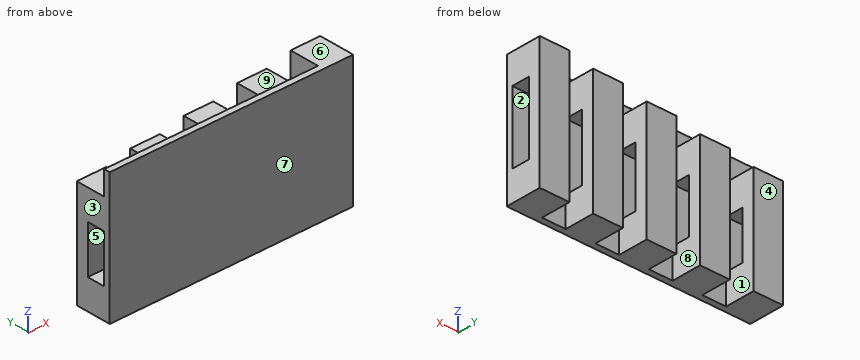
from build123d import *

# Parameters (mm, degrees)
SKETCH1_W            = 41
SKETCH1_H            = 22
BASE_DEPTH           = 1
SKETCH2_W            = 5
SKETCH2_H            = 5
LEGS_EXTRUSION_DEPTH = 5
SKETCH3_W            = 5
SKETCH3_H            = 2
BRIDGE1_DEPTH        = 8
SKETCH4_W            = 5
SKETCH4_H            = 2
BRIDGE2_DEPTH        = 9
SKETCH6_W            = 5
SKETCH6_H            = 2
BRIDGE3_DEPTH        = 10
SKETCH7_W            = 5
SKETCH7_H            = 2
BRIDGE4_DEPTH        = 11
SKETCH8_W            = 5
SKETCH8_H            = 2
BRIDGE5_DEPTH        = 12


with BuildPart() as part:
    # Sketch1 → Base (new body)
    with BuildSketch(Plane(origin=(0, 0, 0), x_dir=(1, 0, 0), z_dir=(0, 1, 0))):
        with Locations((20.5, 11)):
            Rectangle(SKETCH1_W, SKETCH1_H)
    extrude(amount=BASE_DEPTH)

    # Sketch2 → Legs_Extrusion (add)
    with BuildSketch(Plane(origin=(0, 1, 0), x_dir=(1, 0, 0), z_dir=(0, 1, 0))):
        with Locations((2.5, 19.5)):
            Rectangle(SKETCH2_W, SKETCH2_H)
        with Locations((2.5, 6.5)):
            Rectangle(SKETCH2_W, SKETCH2_H)
        with Locations((38.5, 2.5)):
            Rectangle(SKETCH2_W, SKETCH2_H)
        with Locations((38.5, 19.5)):
            Rectangle(SKETCH2_W, SKETCH2_H)
        with Locations((11.5, 19.5)):
            Rectangle(SKETCH2_W, SKETCH2_H)
        with Locations((11.5, 5.5)):
            Rectangle(SKETCH2_W, SKETCH2_H)
        with Locations((20.5, 19.5)):
            Rectangle(SKETCH2_W, SKETCH2_H)
        with Locations((29.5, 19.5)):
            Rectangle(SKETCH2_W, SKETCH2_H)
        with Locations((20.5, 4.5)):
            Rectangle(SKETCH2_W, SKETCH2_H)
        with Locations((29.5, 3.5)):
            Rectangle(SKETCH2_W, SKETCH2_H)
    extrude(amount=LEGS_EXTRUSION_DEPTH)

    # Sketch3 → bridge1 (add)
    with BuildSketch(Plane.XY.offset(-17)):
        with Locations((2.5, 5)):
            Rectangle(SKETCH3_W, SKETCH3_H)
    extrude(amount=BRIDGE1_DEPTH)

    # Sketch4 → bridge2 (add)
    with BuildSketch(Plane.XY.offset(-17)):
        with Locations((11.5, 5)):
            Rectangle(SKETCH4_W, SKETCH4_H)
    extrude(amount=BRIDGE2_DEPTH)

    # Sketch6 → bridge3 (add)
    with BuildSketch(Plane.XY.offset(-17)):
        with Locations((20.5, 5)):
            Rectangle(SKETCH6_W, SKETCH6_H)
    extrude(amount=BRIDGE3_DEPTH)

    # Sketch7 → bridge4 (add)
    with BuildSketch(Plane.XY.offset(-17)):
        with Locations((29.5, 5)):
            Rectangle(SKETCH7_W, SKETCH7_H)
    extrude(amount=BRIDGE4_DEPTH)

    # Sketch8 → bridge5 (add)
    with BuildSketch(Plane.XY.offset(-17)):
        with Locations((38.5, 5)):
            Rectangle(SKETCH8_W, SKETCH8_H)
    extrude(amount=BRIDGE5_DEPTH)


solid = part.part
Work out the finished part from the listing and answer in its coordinate system (mm). Face numbers are marked on the shaded views. A direction names the side the tool comes from. Coordinates: 2 decimals unless noted, no trailing zeros. Order: outer loops, then holes, each group sorted by start corner. A loop starts at its lowest first (then second) coordinate and runs counter-clockwise, first axis right, second up. Notation, with made-up numbers: (0.25, 66) - (21.25, 66) arc R14 cw to (21.25, 91) - close; hole circle Ø8 at (81.25, 80). An arc over 180 degrees is marked (long way). Put each result on its own line as item: value. Start each with the question number.
1) Flat-ended cylindrical pins translate along their axes: pin 1 (1.5 mm diameter, centred on x = 2, y = 2, fed in from +Z); pin 2 (2 mm diameter, centred on x = 24.5, z = -10.5, fed in from +Y); pin 3 (1.5 mm diameter, centred on x = 12.5, y = 2.5, fed in from +Z). Find the tip coordinate at first contact, or state that the pin passes through.
2) Find section B-B (x = 11). Give the vertices of the cut face in (y, z), plus the area to 3 significant figures.
3) Find the intervals of material crossed by line 1 (X direction, y = 4.45, z = -19.75); line 2 (Z direction, x = 9.5, y = 1.2); line 3 (Z direction, x = 20.5, y = 2.55), in increasing order. Write a range as from..to.
4) Find section C-C (z = -8.5). Give the vertices of the cut face in (x, y), plus the area to 3 significant figures.
5) Find section D-D (y = 4.8). Give the vertices of the cut face in (x, z).
6) For a pull along X with two mould halves and no side action, classify the marked faces 1, 2, 3 and 4 as released by +X, released by -X, zero draft, split by the parting line, or undercut.
7) Find section A-A (z = -16). Give the vertices of the cut face in (x, y), plus the area to 3 significant figures.
8) For the marked faces 5, 6, 7, 8 and 9, determine the directions among +Z, -Z, +X, -X, +Y, -Y from which every point of the face is accessible in a straight line to the end or side of a thin tool.
Results list:
1. pin 1: stops at z = -4
1. pin 2: stops at y = 1
1. pin 3: stops at z = -3
2. outline: (0, -22) - (6, -22) - (6, -3) - (1, -3) - (1, 0) - (0, 0) - close; hole (1, -17) - (4, -17) - (4, -8) - (1, -8) - close
2. area: 90.0 mm^2
3. line 1: x = 0..5, 9..14, 18..23, 27..32, 36..41
3. line 2: z = -22..-17, -8..-3
3. line 3: z = -22..-17, -7..-2
4. outline: (0, 0) - (41, 0) - (41, 1) - (5, 1) - (5, 6) - (0, 6) - close; (9, 4) - (14, 4) - (14, 6) - (9, 6) - close; (18, 4) - (23, 4) - (23, 6) - (18, 6) - close; (27, 4) - (32, 4) - (32, 6) - (27, 6) - close; (36, 4) - (41, 4) - (41, 6) - (36, 6) - close
4. area: 106 mm^2
5. outline: (0, -22) - (5, -22) - (5, -4) - (0, -4) - close; (9, -22) - (14, -22) - (14, -3) - (9, -3) - close; (18, -22) - (23, -22) - (23, -2) - (18, -2) - close; (27, -22) - (32, -22) - (32, -1) - (27, -1) - close; (36, -22) - (41, -22) - (41, 0) - (36, 0) - close
6. face 1: undercut
6. face 2: undercut
6. face 3: released by -X
6. face 4: zero draft
7. outline: (0, 0) - (41, 0) - (41, 1) - (0, 1) - close; (0, 4) - (5, 4) - (5, 6) - (0, 6) - close; (9, 4) - (14, 4) - (14, 6) - (9, 6) - close; (18, 4) - (23, 4) - (23, 6) - (18, 6) - close; (27, 4) - (32, 4) - (32, 6) - (27, 6) - close; (36, 4) - (41, 4) - (41, 6) - (36, 6) - close
7. area: 91.0 mm^2
8. face 5: +X, -X
8. face 6: +Z, +X, -X, +Y, -Y
8. face 7: +Z, -Z, +X, -X, -Y
8. face 8: +Z, -Z, +Y
8. face 9: +Z, -X, +Y
